from build123d import *

# Parameters (mm, degrees)
SKETCH1_R           = 21.59
SKETCH1_R_2         = 11.43
SKETCH1_R_3         = 1.217304979
BOSS_EXTRUDE1_DEPTH = 2.54


with BuildPart() as part:
    # Sketch1 → Boss-Extrude1 (new body)
    with BuildSketch(Plane(origin=(0, 0, 0), x_dir=(1, 0, 0), z_dir=(0, 1, 0))):
        with Locations(Location((-126.227589866, 73.421482023, 0), (0, 0, 270))):  # turned: the seam where the file's is
            Circle(SKETCH1_R)
        with Locations(Location((-126.227589866, 73.421482023, 0), (0, 0, 270))):  # turned: the seam where the file's is
            Circle(SKETCH1_R_2, mode=Mode.SUBTRACT)
        with Locations(Location((-126.227589866, 92.001159833, 0), (0, 0, 270))):  # turned: the seam where the file's is
            Circle(SKETCH1_R_3, mode=Mode.SUBTRACT)
        with Locations(Location((-110.137116889, 64.131643118, 0), (0, 0, 270))):  # turned: the seam where the file's is
            Circle(SKETCH1_R_3, mode=Mode.SUBTRACT)
        with Locations(Location((-142.318062844, 64.131643118, 0), (0, 0, 270))):  # turned: the seam where the file's is
            Circle(SKETCH1_R_3, mode=Mode.SUBTRACT)
        with BuildLine():
            Line((-124.112850648, 88.468633425), (-124.473677215, 85.901218995))
            ThreePointArc((-124.473677215, 85.901218995), (-115.31360648, 79.722673269), (-114.542864291, 68.700546449))
            Line((-114.542864291, 68.700546449), (-112.139004888, 67.729324207))
            ThreePointArc((-112.139004888, 67.729324207), (-113.068309283, 81.01899621), (-124.112850648, 88.468633425))
        make_face(mode=Mode.SUBTRACT)
        with BuildLine():
            Line((-119.418746821, 91.635534611), (-120.038701331, 89.576664888))
            ThreePointArc((-120.038701331, 89.576664888), (-121.618568384, 88.728048279), (-122.467184992, 90.307915332))
            Line((-122.467184992, 90.307915332), (-121.847230483, 92.366785055))
            ThreePointArc((-121.847230483, 92.366785055), (-120.26736343, 93.215401663), (-119.418746821, 91.635534611))
        make_face(mode=Mode.SUBTRACT)
        with BuildLine():
            Line((-115.121572952, 89.382949486), (-116.231928828, 87.541646155))
            ThreePointArc((-116.231928828, 87.541646155), (-117.972703409, 87.110561582), (-118.403787983, 88.851336163))
            Line((-118.403787983, 88.851336163), (-117.293432106, 90.692639495))
            ThreePointArc((-117.293432106, 90.692639495), (-115.552657525, 91.123724068), (-115.121572952, 89.382949486))
        make_face(mode=Mode.SUBTRACT)
        with BuildLine():
            Line((-111.515818176, 86.136663069), (-113.047448813, 84.627558791))
            ThreePointArc((-113.047448813, 84.627558791), (-114.840756806, 84.640843967), (-114.827471629, 86.43415196))
            Line((-114.827471629, 86.43415196), (-113.295840992, 87.943256238))
            ThreePointArc((-113.295840992, 87.943256238), (-111.502532999, 87.929971061), (-111.515818176, 86.136663069))
        make_face(mode=Mode.SUBTRACT)
        with BuildLine():
            Line((-108.825963306, 82.098777014), (-110.683515106, 81.01582298))
            ThreePointArc((-110.683515106, 81.01582298), (-112.417711859, 81.472650821), (-111.960884018, 83.206847573))
            Line((-111.960884018, 83.206847573), (-110.103332218, 84.289801607))
            ThreePointArc((-110.103332218, 84.289801607), (-108.369135466, 83.832973767), (-108.825963306, 82.098777014))
        make_face(mode=Mode.SUBTRACT)
        with BuildLine():
            Line((-107.219468651, 77.520675013), (-109.287297384, 76.931291893))
            ThreePointArc((-109.287297384, 76.931291893), (-110.854418289, 77.803222004), (-109.982488178, 79.37034291))
            Line((-109.982488178, 79.37034291), (-107.914659445, 79.95972603))
            ThreePointArc((-107.914659445, 79.95972603), (-106.34753854, 79.087795919), (-107.219468651, 77.520675013))
        make_face(mode=Mode.SUBTRACT)
        with BuildLine():
            Line((-106.796348562, 72.687372581), (-108.945718941, 72.628253164))
            ThreePointArc((-108.945718941, 72.628253164), (-110.24820091, 73.861002437), (-109.015451637, 75.163484407))
            Line((-109.015451637, 75.163484407), (-106.866081259, 75.222603824))
            ThreePointArc((-106.866081259, 75.222603824), (-105.563599289, 73.989854551), (-106.796348562, 72.687372581))
        make_face(mode=Mode.SUBTRACT)
        with BuildLine():
            Line((-107.582944914, 67.899773058), (-109.680045174, 68.374597899))
            ThreePointArc((-109.680045174, 68.374597899), (-110.63680055, 69.891419972), (-109.119978476, 70.848175348))
            Line((-109.119978476, 70.848175348), (-107.022878216, 70.373350508))
            ThreePointArc((-107.022878216, 70.373350508), (-106.06612284, 68.856528434), (-107.582944914, 67.899773058))
        make_face(mode=Mode.SUBTRACT)
        with BuildLine():
            Line((-138.201435626, 64.066488437), (-136.158402791, 65.662680625))
            ThreePointArc((-136.158402791, 65.662680625), (-126.227589866, 60.819099531), (-116.296776942, 65.662680625))
            Line((-116.296776942, 65.662680625), (-114.253744106, 64.066488437))
            ThreePointArc((-114.253744106, 64.066488437), (-126.227589866, 58.226453649), (-138.201435626, 64.066488437))
        make_face(mode=Mode.SUBTRACT)
        with BuildLine():
            Line((-113.858179141, 58.417824681), (-115.331235369, 59.984155898))
            ThreePointArc((-115.331235369, 59.984155898), (-115.276225385, 61.776669204), (-113.483712078, 61.721659219))
            Line((-113.483712078, 61.721659219), (-112.01065585, 60.155328003))
            ThreePointArc((-112.01065585, 60.155328003), (-112.065665835, 58.362814697), (-113.858179141, 58.417824681))
        make_face(mode=Mode.SUBTRACT)
        with BuildLine():
            Line((-117.957562018, 55.822655508), (-118.996999541, 57.70490357))
            ThreePointArc((-118.996999541, 57.70490357), (-118.499942442, 59.428000866), (-116.776845146, 58.930943767))
            Line((-116.776845146, 58.930943767), (-115.737407623, 57.048695705))
            ThreePointArc((-115.737407623, 57.048695705), (-116.234464722, 55.325598409), (-117.957562018, 55.822655508))
        make_face(mode=Mode.SUBTRACT)
        with BuildLine():
            Line((-122.571805912, 54.323123481), (-123.112913235, 56.404106661))
            ThreePointArc((-123.112913235, 56.404106661), (-122.204753938, 57.950514351), (-120.658346248, 57.042355055))
            Line((-120.658346248, 57.042355055), (-120.117238925, 54.961371875))
            ThreePointArc((-120.117238925, 54.961371875), (-121.025398222, 53.414964185), (-122.571805912, 54.323123481))
        make_face(mode=Mode.SUBTRACT)
        with BuildLine():
            Line((-127.413645248, 54.012583859), (-127.422735052, 56.162747924))
            ThreePointArc((-127.422735052, 56.162747924), (-126.16001216, 57.436192446), (-124.886567638, 56.173469555))
            Line((-124.886567638, 56.173469555), (-124.877477834, 54.02330549))
            ThreePointArc((-124.877477834, 54.02330549), (-126.140200725, 52.749860968), (-127.413645248, 54.012583859))
        make_face(mode=Mode.SUBTRACT)
        with BuildLine():
            Line((-132.181645209, 54.910369677), (-131.658151598, 56.99585345))
            ThreePointArc((-131.658151598, 56.99585345), (-130.119477518, 57.91705491), (-129.198276059, 56.37838083))
            Line((-129.198276059, 56.37838083), (-129.72176967, 54.292897057))
            ThreePointArc((-129.72176967, 54.292897057), (-131.26044375, 53.371695598), (-132.181645209, 54.910369677))
        make_face(mode=Mode.SUBTRACT)
        with BuildLine():
            Line((-136.578967944, 56.960588147), (-135.555481672, 58.851557206))
            ThreePointArc((-135.555481672, 58.851557206), (-133.8366485, 59.363165043), (-133.325040663, 57.644331871))
            Line((-133.325040663, 57.644331871), (-134.348526935, 55.753362813))
            ThreePointArc((-134.348526935, 55.753362813), (-136.067360107, 55.241754975), (-136.578967944, 56.960588147))
        make_face(mode=Mode.SUBTRACT)
        with BuildLine():
            Line((-140.331852578, 60.035600332), (-138.872092074, 61.614330011))
            ThreePointArc((-138.872092074, 61.614330011), (-137.080107937, 61.684493435), (-137.009944513, 59.892509298))
            Line((-137.009944513, 59.892509298), (-138.469705017, 58.313779619))
            ThreePointArc((-138.469705017, 58.313779619), (-140.261689154, 58.243616195), (-140.331852578, 60.035600332))
        make_face(mode=Mode.SUBTRACT)
        with BuildLine():
            Line((-128.342329084, 88.468633425), (-127.981502517, 85.901218995))
            ThreePointArc((-127.981502517, 85.901218995), (-137.141573252, 79.722673269), (-137.912315442, 68.700546449))
            Line((-137.912315442, 68.700546449), (-140.316174844, 67.729324207))
            ThreePointArc((-140.316174844, 67.729324207), (-139.386870449, 81.01899621), (-128.342329084, 88.468633425))
        make_face(mode=Mode.SUBTRACT)
        with BuildLine():
            Line((-145.405843636, 70.211086776), (-143.312832898, 70.703625283))
            ThreePointArc((-143.312832898, 70.703625283), (-141.78797583, 69.759728585), (-142.731872528, 68.234871518))
            Line((-142.731872528, 68.234871518), (-144.824883266, 67.742333011))
            ThreePointArc((-144.824883266, 67.742333011), (-146.349740334, 68.686229709), (-145.405843636, 70.211086776))
        make_face(mode=Mode.SUBTRACT)
        with BuildLine():
            Line((-145.603634629, 75.058841074), (-143.45384123, 75.017896343))
            ThreePointArc((-143.45384123, 75.017896343), (-142.210123747, 73.72588362), (-143.502136471, 72.482166138))
            Line((-143.502136471, 72.482166138), (-145.65192987, 72.523110869))
            ThreePointArc((-145.65192987, 72.523110869), (-146.895647352, 73.815123592), (-145.603634629, 75.058841074))
        make_face(mode=Mode.SUBTRACT)
        with BuildLine():
            Line((-144.595145511, 79.804659518), (-142.522407551, 79.232780616))
            ThreePointArc((-142.522407551, 79.232780616), (-141.637258855, 77.67308775), (-143.196951721, 76.787939054))
            Line((-143.196951721, 76.787939054), (-145.269689681, 77.359817956))
            ThreePointArc((-145.269689681, 77.359817956), (-146.154838377, 78.919510823), (-144.595145511, 79.804659518))
        make_face(mode=Mode.SUBTRACT)
        with BuildLine():
            Line((-142.443161045, 84.153085195), (-140.57651944, 83.085875164))
            ThreePointArc((-140.57651944, 83.085875164), (-140.105045579, 81.355602801), (-141.835317942, 80.88412894))
            Line((-141.835317942, 80.88412894), (-143.701959547, 81.951338971))
            ThreePointArc((-143.701959547, 81.951338971), (-144.173433408, 83.681611334), (-142.443161045, 84.153085195))
        make_face(mode=Mode.SUBTRACT)
        with BuildLine():
            Line((-139.281655738, 87.833401378), (-137.737320617, 86.337300725))
            ThreePointArc((-137.737320617, 86.337300725), (-137.708873791, 84.544169154), (-139.502005362, 84.515722328))
            Line((-139.502005362, 84.515722328), (-141.046340483, 86.011822981))
            ThreePointArc((-141.046340483, 86.011822981), (-141.074787309, 87.804954552), (-139.281655738, 87.833401378))
        make_face(mode=Mode.SUBTRACT)
        with BuildLine():
            Line((-135.307453093, 90.61648534), (-134.181568986, 88.784635699))
            ThreePointArc((-134.181568986, 88.784635699), (-134.597920188, 87.040278588), (-136.342277299, 87.45662979))
            Line((-136.342277299, 87.45662979), (-137.468161405, 89.288479432))
            ThreePointArc((-137.468161405, 89.288479432), (-137.051810203, 91.032836542), (-135.307453093, 90.61648534))
        make_face(mode=Mode.SUBTRACT)
        with BuildLine():
            Line((-130.767972107, 92.329072679), (-130.130632351, 90.275518159))
            ThreePointArc((-130.130632351, 90.275518159), (-130.965861112, 88.688532661), (-132.552846609, 89.523761422))
            Line((-132.552846609, 89.523761422), (-133.190186365, 91.577315942))
            ThreePointArc((-133.190186365, 91.577315942), (-132.354957605, 93.164301439), (-130.767972107, 92.329072679))
        make_face(mode=Mode.SUBTRACT)
    extrude(amount=BOSS_EXTRUDE1_DEPTH)


solid = part.part
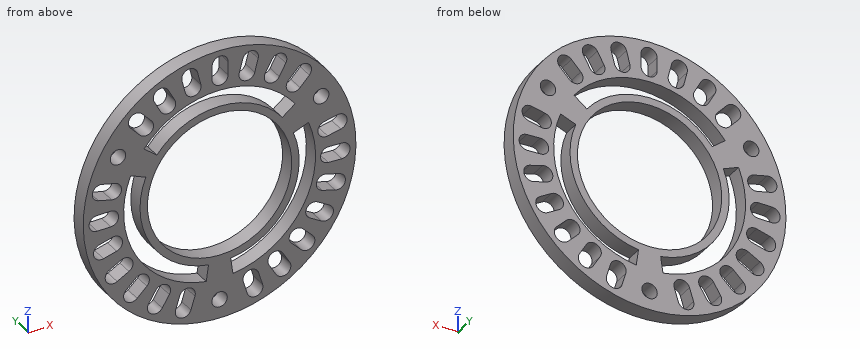
Check sheet for the modelled part. Datum: model origin and axes. Units: mm. Give positions to 0.01 mm unless a question says otherwise; leave off trailing zeros. Write each loop counter-clockwise with the first axis right and the second up, starting at its lowest first coordinate (ties: lowest second). Pieces come first, ordered by that corner, then holes. Notation, with made-up numbers: M 71,18.25 L 81,18.25 A33 cw 81,48.25 Z; hole C 46.25,3 d9. An arc over 180 degrees is marked long. Use one line per item in the form item = value.
(1) Depth check by flat-ended pin: P1, Ø1.5, axis at y = 2, z = -86, coming from the -X side; P2, Ø3, axis at x = -126.23, z = -92, coming from the -Y side. Enter the tip coordinate at first touch or a pass-through.
Answer block:
P1 = -144.29
P2 = 0
(2) Section check B-B on y = 0.95. State how many separate pieces and enclosed holes the cut face has, plus the area to 3 significant figures.
Answer block:
separate_pieces = 1
enclosed_holes = 28
area = 623 mm2
(3) Section check A-A on z = -76. Record the boundary of the cut face in (x, y), plus the area to 3 significant figures.
Answer block:
outline = M -147.66,0 L -141.2,0 L -141.2,2.54 L -147.66,2.54 Z; M -138.56,0 L -137.36,0 L -137.36,2.54 L -138.56,2.54 Z; M -115.09,0 L -113.89,0 L -113.89,2.54 L -115.09,2.54 Z; M -111.25,0 L -104.79,0 L -104.79,2.54 L -111.25,2.54 Z
area = 38.9 mm2
(4) Material ranges on line 1 along Z through (x, y) = (-107, 1.3); line 2 along X through (y, z) = (2.25, -85); line 3 along X through (y, z) = (0.5, -76.5), recorded low to high.
Answer block:
line_1 = -83.24 to -79.87, -77.61 to -75.22, -72.68 to -70.37, -67.91 to -63.6
line_2 = -144.45 to -140, -137.43 to -136.07, -131.2 to -121.25, -116.39 to -115.09, -112.67 to -108
line_3 = -147.6 to -141.11, -138.45 to -137.24, -115.22 to -114.01, -111.35 to -104.86
